from build123d import *

# Parameters (mm, degrees)
BOSS_EXTRUDE1_DEPTH = 6.35
BOSS_EXTRUDE2_DEPTH = 6.35
BOSS_EXTRUDE2_DRAFT = 63
CUT_EXTRUDE1_DEPTH  = 63.5
SKETCH4_R           = 7.9375
CUT_EXTRUDE2_DEPTH  = 254


with BuildPart() as part:
    # Sketch1 → Boss-Extrude1 (new body)
    with BuildSketch(Plane.XY):
        with BuildLine():
            Line((-68.693731343, 19.059477612), (51.956268657, 19.059477612))
            Line((51.956268657, 19.059477612), (51.956268657, -44.440522388))
            Line((51.956268657, -44.440522388), (-68.693731343, -44.440522388))
            ThreePointArc((-68.693731343, -44.440522388), (-100.443731343, -12.690522388), (-68.693731343, 19.059477612))
        make_face()
    extrude(amount=BOSS_EXTRUDE1_DEPTH)


with BuildPart() as boss_extrude2_tool:
    # 3DSketch1 → Boss-Extrude2 (with draft: the straight prism first)
    with BuildSketch(Plane(origin=(-68.627300229, -31.913895704, 12.7), x_dir=(0.9191450300180579, 0.39391929857916763, 0), z_dir=(0, 0, 1))):
        with BuildLine():
            Line((0, 0), (81.711993169, -35.019425644))
            Line((81.711993169, -35.019425644), (96.720318444, 0))
            Line((96.720318444, 0), (15.008325276, 35.019425644))
            ThreePointArc((15.008325276, 35.019425644), (-10.005550184, 25.01387546), (0, 0))
        make_face()
    extrude(amount=-BOSS_EXTRUDE2_DEPTH)
    # Boss-Extrude2: the draft: its side faces are tilted about the plane it starts from
    boss_extrude2_sides = [boss_extrude2_tool.faces().sort_by_distance(p)[0] for p in [
        (-87.677300229, -12.863895704, 9.525),
        (-24.177300229, -31.913895704, 9.525),
        (20.272699771, -12.863895704, 9.525),
        (-24.177300229, 6.186104296, 9.525),
    ]]
    draft(boss_extrude2_sides, Plane(origin=(-68.627300229, -31.913895704, 12.7), x_dir=(0.9191450300180579, 0.39391929857916763, 0), z_dir=(0, 0, 1)), BOSS_EXTRUDE2_DRAFT)


with BuildPart() as part_1:
    add(part.part)

    # Boss-Extrude2: add boss_extrude2_tool
    add(boss_extrude2_tool.part)

    # Sketch3 → Cut-Extrude1 (cut)
    with BuildSketch(Plane.XZ.offset(44.440522388)):
        Polygon((32.598411505, 6.35), (51.956268657, 3.175), (51.956268657, 6.35), align=None)
    extrude(amount=-CUT_EXTRUDE1_DEPTH, mode=Mode.SUBTRACT)

    # Sketch4 → Cut-Extrude2 (cut)
    with BuildSketch(Plane.XY.offset(12.7)):
        with Locations((-68.627300229, -12.863895704)):
            Circle(SKETCH4_R)
        with Locations((-43.227300229, -12.863895704)):
            Circle(SKETCH4_R)
        with Locations((-17.827300229, -12.863895704)):
            Circle(SKETCH4_R)
        with Locations((7.572699771, -12.863895704)):
            Circle(SKETCH4_R)
    extrude(amount=-CUT_EXTRUDE2_DEPTH, mode=Mode.SUBTRACT)


solid = part_1.part
Input: part model. Units: mm. Frame: model coordinates. Coordinates: 2 decimals unless noted, no trailing zeros. Write each loop counter-clockwise with the first axis right and the second up, starting at its lowest first coordinate (ties: lowest second). Pieces come first, ordered by that corner, then holes. Notation, with made-up numbers: M -1.75,63.25 L 57.25,63.25 A22 cw 57.25,84.25 Z; hole C 53,52.25 d9. An arc over 180 degrees is marked long. Answer as a JSON object with one key per item and string values. Group by question number.
(1) Section C-C on x = 1.5. Output: boundary loops of the cut face in (y, z).
(2) Section D-D on y = -18.5. Give the number of separate pieces and of enclosed holes in the cut face, plus the area to 3 significant figures.
(3) Section B-B on x = -32.5. Output: boundary loops of the cut face in (y, z), plus the area to 3 significant figures.
(4) Ray query, line 1 along X through (y, z) = (-18, 6.5); line 2 along X through (y, z) = (-16, 9.75); line 3 along Y through (x, z) = (-22, 6.25). Return the intervals inside material, ascending. Write a range as [from, to].
(5) Mould query, pull axis X, two halves, no side actions, for faces 1 (the face through (-18.66, -38.06, 9.57)), 2 (the face through (1.27, -17.69, 6.44)), 3 (the face through (51.956, -12, 2)). Classes: pulls with the +X half, pulls with the -X half, needs draft (parallel to the pull), parting line crosses it, or undercut.
(6) Contact query for flat-ended pins moving along their axis: P1, Ø14.5, axis at x = 7.57, y = -12.86, coming from the +Z side; P2, Ø4, axis at x = -13.5, y = 6.5, coming from the -Z side; P3, Ø6, axis at x = -73, z = 9, coming from the +Y side; P4, Ø1.5, axis at x = -33, z = 11, coming from the -Y side. Output: stop coordinate, or through.
(7) Section A-A on z = 11. Output: boundary loops of the cut face in (x, y) (1 decimal).
Result set:
{
 "1": {"outline": "M -44.44,0 L -17.98,0 L -17.98,12.7 L -31.91,12.7 L -44.38,6.35 L -44.44,6.35 Z; M -7.75,0 L 19.06,0 L 19.06,6.35 L 18.65,6.35 L 6.19,12.7 L -7.75,12.7 Z"},
 "2": {"separate pieces": "5", "enclosed holes": "0", "area": "1,130 mm2"},
 "3": {"outline": "M -44.44,0 L 19.06,0 L 19.06,6.35 L 18.65,6.35 L 6.19,12.7 L -31.91,12.7 L -44.38,6.35 L -44.44,6.35 Z", "area": "724 mm2"},
 "4": {"line 1": "x = [-99.42, -74.68], [-62.58, -49.28], [-37.18, -23.88], [-11.78, 1.52], [13.62, 32.44]", "line 2": "x = [-93.27, -75.92], [-61.34, -50.52], [-35.94, -25.12], [-10.54, 0.28], [14.86, 26.06]", "line 3": "y = [-44.44, -19.62], [-6.11, 19.06]"},
 "5": {"face 1": "needs draft", "face 2": "undercut", "face 3": "pulls with the +X half"},
 "6": {"P1": "passes through", "P2": "stops at z = 0", "P3": "stops at y = 18.93", "P4": "stops at y = -36.72"},
 "7": {"outline": "M -68.6,-35.3 L 23.6,-35.3 L 23.6,9.5 L -68.6,9.5 A22.4 ccw Z; hole C -68.6,-12.9 d15.9; hole C -43.2,-12.9 d15.9; hole C -17.8,-12.9 d15.9; hole C 7.6,-12.9 d15.9"}
}
